The listing builds one solid part. Answer for the finished solid, in the listing's coordinates (mm). Coordinates: 2 decimals unless noted, no trailing zeros. Write each loop counter-clockwise with the first axis right and the second up, starting at its lowest first coordinate (ties: lowest second). Pieces come first, ordered by that corner, then holes.
from build123d import *

# Parameters (mm, degrees)
F1_DEPTH = 3.81
F3_DEPTH = 113.03
F4_W     = 102.2572831413
F4_H     = 63.9604873323
F4_H_2   = 99.7172831413
F5_DEPTH = 76.2
F6_DEPTH = 1.778


with BuildPart() as f1:
    # F0 (on Front) → F1 (new body)
    with BuildSketch(Plane.XZ):
        with BuildLine():
            Line((-61.7348178759, 19.6423271978), (-64.2748178759, 19.6423271978))
            Line((-64.2748178759, 19.6423271978), (-64.2748178759, 17.1023271978))
            Line((-64.2748178759, 17.1023271978), (-64.2748178759, 6.9423271978))
            ThreePointArc((-64.2748178759, 6.9423271978), (-54.844956833, -10.8368491458), (-36.0173178759, -17.9460967888))
            ThreePointArc((-36.0173178759, -17.9460967888), (-17.1896789189, -10.8368491458), (-7.7598178759, 6.9423271978))
            ThreePointArc((-7.7598178759, 6.9423271978), (0.406829165, -9.8369400067), (17.212230035, -17.9496728022))
            Line((17.212230035, -17.9496728022), (20.4976821241, -17.9496728022))
            Line((20.4976821241, -17.9496728022), (23.7831342132, -17.9496728022))
            ThreePointArc((23.7831342132, -17.9496728022), (40.5885350832, -9.8369400067), (48.7551821241, 6.9423271978))
            Line((48.7551821241, 6.9423271978), (48.7551821241, 17.1023271978))
            Line((48.7551821241, 17.1023271978), (48.7551821241, 19.6423271978))
            Line((48.7551821241, 19.6423271978), (46.2151821241, 19.6423271978))
            Line((46.2151821241, 19.6423271978), (-61.7348178759, 19.6423271978))
        make_face()
        with BuildLine():
            ThreePointArc((46.2151821241, 6.9423271978), (20.4976821241, -15.5999571068), (-5.2198178759, 6.9423271978))
            ThreePointArc((-5.2198178759, 6.9423271978), (-4.3618373454, 12.4360262368), (-1.3381814351, 17.1023271978))
            Line((-1.3381814351, 17.1023271978), (41.7701821241, 17.1023271978))
            ThreePointArc((41.7701821241, 17.1023271978), (44.9132717665, 15.8004168402), (46.2151821241, 12.6573271978))
            Line((46.2151821241, 12.6573271978), (46.2151821241, 6.9423271978))
        make_face(mode=Mode.SUBTRACT)
        with BuildLine():
            ThreePointArc((-14.3130178759, 17.1023271978), (-11.2183816966, 12.4521014886), (-10.2998178759, 6.9423271978))
            ThreePointArc((-10.2998178759, 6.9423271978), (-36.010114835, -15.409671479), (-61.7348178759, 6.9257458672))
            Line((-61.7348178759, 6.9257458672), (-61.7348178759, 12.6573271978))
            ThreePointArc((-61.7348178759, 12.6573271978), (-60.4329075183, 15.8004168402), (-57.2898178759, 17.1023271978))
            Line((-57.2898178759, 17.1023271978), (-14.3130178759, 17.1023271978))
        make_face(mode=Mode.SUBTRACT)
    extrude(amount=F1_DEPTH)

    # F2 (on face) → F3 (join)
    with BuildSketch(Plane.YZ.offset(48.7551821241)):
        with BuildLine():
            Line((-3.81, 14.5623271978), (-3.81, 19.6423271978))
            Line((-3.81, 19.6423271978), (-105.41, 19.6423271978))
            ThreePointArc((-105.41, 19.6423271978), (-122.7306756991, 14.2570441707), (-133.9442287254, 0))
            ThreePointArc((-133.9442287254, 0), (-131.4042287254, -2.8934895881), (-128.8642287254, 0))
            ThreePointArc((-128.8642287254, 0), (-119.2136428029, 10.6256409156), (-105.41, 14.5623271978))
            Line((-105.41, 14.5623271978), (-3.81, 14.5623271978))
        make_face()
    extrude(amount=-F3_DEPTH)

    # F4 (on face) → F5 (cut)
    with BuildSketch(Plane.XY.offset(19.6423271978)):
        with Locations((-7.4534594466, -137.3902436662)):
            Rectangle(F4_W, F4_H)
        with Locations((-7.4534594466, -55.5513584293)):
            Rectangle(F4_W, F4_H_2)
    extrude(amount=-F5_DEPTH, mode=Mode.SUBTRACT)

    # F6 (cut): a face of the model
    f6_faces = [f1.faces().sort_by_distance(p)[0] for p in [
        (-7.4534594466, -5.6927168587, 17.1023271978),
    ]]
    extrude(f6_faces, amount=-F6_DEPTH, mode=Mode.SUBTRACT)


solid = f1.part
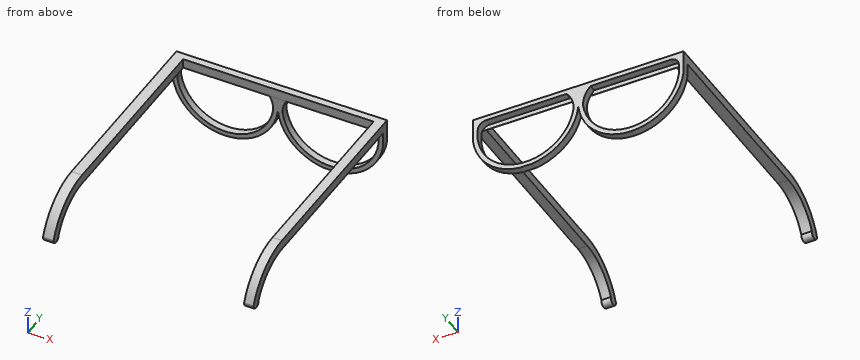
Q1. The part is cut by section C-C, the plane z = -4.5. Write down the section's boundary in (x, y).
Answers below:
outline: (-60.21, -3.81) - (-57.18, -3.81) - (-57.18, 0) - (-60.21, 0) - close; (-14.86, -3.81) - (-11.83, -3.81) - (-11.83, 0) - (-14.86, 0) - close; (-3.8, -3.81) - (-0.78, -3.81) - (-0.78, 0) - (-3.8, 0) - close; (41.77, -3.81) - (44.79, -3.81) - (44.79, 0) - (41.77, 0) - close
Q2. The part is cut by section A-A, the plane y = -40.5. Write down the section's boundary in (x, z), then the cut area to 3 significant figures.
Answers below:
outline: (-64.27, 14.56) - (-58.58, 14.56) - (-58.58, 19.64) - (-64.27, 19.64) - close; (43.68, 14.56) - (48.76, 14.56) - (48.76, 19.64) - (43.68, 19.64) - close
area: 54.7 mm2
Q3. Find the intervals of material crossed by probe 1 along X at (y, z) = (-67.5, 15); probe 2 along Z at (x, y) = (44.5, -13.5), in increasing order.
Answers below:
probe 1: x = -64.27 to -58.58, 43.68 to 48.76
probe 2: z = 14.56 to 19.64
Q4. Given pin 1 (4 mm diameter, centred on x = -25.5, y = -1, fed in from -Z); pin 2 (0.8 mm diameter, centred on x = -41.5, z = 16.5, fed in from +Y); pin 3 (10 mm diameter, centred on y = -114, z = 7, fed in from -X); pin 4 (2.5 mm diameter, centred on x = -25.5, z = 17.5, fed in from -Y), each flat-ended and moving along its own axis, determine where each tip first touches the part or whether it passes through.
Answers below:
pin 1: stops at z = -16.64
pin 2: stops at y = -3.81
pin 3: passes through
pin 4: stops at y = -3.91
Q5. The part is cut by section B-B, the plane x = 36.5. Write down the section's boundary in (y, z).
Answers below:
outline: (-3.91, 14.56) - (-3.81, 14.56) - (-3.81, 17.1) - (0, 17.1) - (0, 19.64) - (-3.91, 19.64) - close; (-3.81, -13.21) - (0, -13.21) - (0, -10.08) - (-3.81, -10.08) - close
Q6. The part is cut by section D-D, the plane z = 2.5. Write down the section's boundary in (x, y).
Answers below:
outline: (-64.27, -132.86) - (-58.58, -132.86) - (-58.58, -127.45) - (-64.27, -127.45) - close; (-63.34, -3.81) - (-60.71, -3.81) - (-60.71, 0) - (-63.34, 0) - close; (-11.33, -3.81) - (-8.69, -3.81) - (-8.69, 0) - (-11.33, 0) - close; (-6.87, -3.81) - (-4.23, -3.81) - (-4.23, 0) - (-6.87, 0) - close; (43.68, -132.86) - (48.76, -132.86) - (48.76, -127.45) - (43.68, -127.45) - close; (45.23, -3.81) - (47.86, -3.81) - (47.86, 0) - (45.23, 0) - close
